from build123d import *

# Parameters (mm, degrees)
SKETCH2_R           = 10
BOSS_EXTRUDE1_DEPTH = 10


with BuildPart() as part:
    # Sketch1 → Revolve1 (revolve)
    with BuildSketch(Plane(origin=(0, 0, 0), x_dir=(1, 0, 0), z_dir=(0, 1, 0))):
        Polygon((-50, 50), (-50, -50), (-45, -50), (-40, -50), (-40, -40), (-45, -40), (-45, -25), (-40, -25), (-40, -15), (-45, -15), (-45, 15), (-40, 15), (-40, 25), (-45, 25), (-45, 40), (-40, 40), (-40, 50), (-45, 50), align=None)
    revolve(axis=Axis((0, 0, -100.912408759), (0, 0, 1)))

    # Sketch2 → Boss-Extrude1 (add)
    # profile 1 of 2: a face of its own
    with BuildSketch(Plane.XY.offset(50)):
        with BuildLine():
            Line((45.82575695, 20), (100, 20))
            Line((100, 20), (100, -20))
            Line((100, -20), (45.82575695, -20))
            ThreePointArc((45.82575695, -20), (50, 0), (45.82575695, 20))
        make_face()
        with Locations((80, 0)):
            Circle(SKETCH2_R, mode=Mode.SUBTRACT)
    # profile 2 of 2: a face of its own
    with BuildSketch(Plane.XY.offset(50)):
        with BuildLine():
            Line((-100, 20), (-100, -20))
            Line((-100, -20), (-45.82575695, -20))
            ThreePointArc((-45.82575695, -20), (-50, 0), (-45.82575695, 20))
            Line((-45.82575695, 20), (-100, 20))
        make_face()
        with Locations((-80, 0)):
            Circle(SKETCH2_R, mode=Mode.SUBTRACT)
    boss_extrude1 = extrude(amount=-BOSS_EXTRUDE1_DEPTH)

    # Mirror1: Boss-Extrude1 across plane
    add(boss_extrude1.mirror(Plane.XY))


solid = part.part
Part model, mm, in its own coordinate system. A direction names the side the tool comes from. Coordinates: 2 decimals unless noted, no trailing zeros. Loops run counter-clockwise (first coordinate to the right, second up) from the corner with the lowest first, then second, coordinate; pieces in that order, holes last. Notation, with made-up numbers: M -39.75,64.25 L -11.75,64.25 A31 cw -11.75,102.25 Z; hole C 30.25,-19 d11. An arc over 180 degrees is marked long. Use a Markdown table: item, result. Add a question column.
Q1. Mould opens along X. For faces 1 (the flat face through (100, 0, -45)), 2 (the flat face through (-100, 0, -45)), 3 (the flat face through (-30.2, 26.5, 40)) say: +X half, -X half, draft (parallel to the pull), parting line (faces both ways), or undercut.
Q2. Cut at C-C (z = 23). Write the cut outline in (x, y).
Q3. Probe L1, parallel to Y at x = 0, z = -43; L2, parallel to Y at x = -80, z = -41. List the from-to ranges inside material, lowest first.
Q4. Cut at B-B (x = 57). Write the cut outline in (y, z), and give its area (3 significant figures).
Q5. Pin check, flat tips, straight feed: P1, Ø12, axis at x = -80, y = 0, coming from the +Z side; P2, Ø10, axis at y = 31.5, z = -21.5, coming from the -X side; P3, Ø8, axis at y = 32, z = -12.5, coming from the -X side; P4, Ø2, axis at y = -7.5, z = -11, coming from the -X side. Stop position of each tip, or through.
Q6. Cut at D-D (y = 0). Give the number of separate pieces and of enclosed holes in the cut face, and give its area (3 significant figures).
Q7. Which spindle directions (+Z, -Z, +X, -X, +Y, -Y) get a long thin tool onto all of the face, cutting with end or side? Do faces 4 (the flat face through (73, 20, 45)), 5 (the flat face through (-73, -20, -45)), 6 (the flat face through (-30.2, 26.5, 15)), 7 (the flat face through (-73, 20, 45)). Say none if no direction does.
Q8. Cut at A-A (x = 80). Write the cut outline in (y, z).
Worked out:
| question | item | result |
|---|---|---|
| 1 | face 1 | +X half |
| 1 | face 2 | -X half |
| 1 | face 3 | undercut |
| 2 | outline | C 0,0 d100; hole C 0,0 d80 |
| 3 | L1 | y = -50 to -40, 40 to 50 |
| 3 | L2 | y = -20 to -10, 10 to 20 |
| 4 | outline | M -20,-50 L 20,-50 L 20,-40 L -20,-40 Z; M -20,40 L 20,40 L 20,50 L -20,50 Z |
| 4 | area | 800 mm2 |
| 5 | P1 | passes through |
| 5 | P2 | stops at x = -42.4 |
| 5 | P3 | stops at x = -41.42 |
| 5 | P4 | stops at x = -49.58 |
| 6 | separate pieces | 6 |
| 6 | enclosed holes | 0 |
| 6 | area | 2,600 mm2 |
| 7 | face 4 | +Z, -Z, +X, +Y |
| 7 | face 5 | +Z, -Z, -X, -Y |
| 7 | face 6 | none |
| 7 | face 7 | +Z, -Z, -X, +Y |
| 8 | outline | M -20,-50 L -10,-50 L -10,-40 L -20,-40 Z; M -20,40 L -10,40 L -10,50 L -20,50 Z; M 10,-50 L 20,-50 L 20,-40 L 10,-40 Z; M 10,40 L 20,40 L 20,50 L 10,50 Z |
